Autodesk Inventor part; units mm, degrees
ref_plane "YZ Plane" through (0, 0, 0) normal (1, 0, 0) x (0, 1, 0)
ref_plane "XZ Plane" through (0, 0, 0) normal (0, 1, 0) x (-1, 0, 0)
ref_plane "XY Plane" through (0, 0, 0) normal (0, 0, 1) x (1, 0, 0)
sketch "Sketch4" plane through (0, 0, 0) normal (0, 1, 0) x (-1, 0, 0)
  line L0 (-50.8, 38.1) -> (-50.8, -38.1)
  line L1 (-50.8, -38.1) -> (50.8, -38.1)
  line L2 (50.8, -38.1) -> (50.8, 38.1)
  line L3 (50.8, 38.1) -> (-50.8, 38.1)
  line L4 (-50.8, 38.1) -> (50.8, -38.1) construction
  line L5 (-50.8, -38.1) -> (50.8, 38.1) construction
  point P0 (0, 0)
  dimension "d14" = 76.2
  dimension "d15" = 101.6
extrude "Extrusion4" add sketch "Sketch4" along normal blind 6.35
sketch "Sketch6" plane through (0, 6.35, 0) normal (0, 1, 0) x (1, 0, 0)
  line L0 (-50.8, 38.1) -> (-50.8, -38.1) construction
  line L1 (-50.8, 0) -> (50.8, 0) construction
  line L2 (50.8, -38.1) -> (50.8, 38.1) construction
  line L3 (-50.8, -12.7) -> (-25.4, -12.7)
  line L4 (-25.4, -12.7) -> (-25.4, 12.7)
  line L5 (-25.4, 12.7) -> (-50.8, 12.7)
  line L6 (-50.8, 12.7) -> (-50.8, -12.7)
  line L7 (-50.8, -12.7) -> (-25.4, 12.7) construction
  line L8 (-25.4, -12.7) -> (-50.8, 12.7) construction
  line L9 (-47.625, -9.525) -> (-28.575, -9.525)
  line L10 (-28.575, -9.525) -> (-28.575, 9.525)
  line L11 (-28.575, 9.525) -> (-47.625, 9.525)
  line L12 (-47.625, 9.525) -> (-47.625, -9.525)
  line L13 (-47.625, -9.525) -> (-28.575, 9.525) construction
  line L14 (-28.575, -9.525) -> (-47.625, 9.525) construction
  line L15 (50.8, 38.1) -> (-50.8, 38.1) construction
  line L16 (0, 38.1) -> (0, -38.1) construction
  line L17 (-50.8, -38.1) -> (50.8, -38.1) construction
  line L18 (50.8, -12.7) -> (25.4, -12.7)
  line L19 (25.4, -12.7) -> (25.4, 12.7)
  line L20 (25.4, 12.7) -> (50.8, 12.7)
  line L21 (50.8, 12.7) -> (50.8, -12.7)
  line L22 (47.625, -9.525) -> (28.575, -9.525)
  line L23 (28.575, -9.525) -> (28.575, 9.525)
  line L24 (28.575, 9.525) -> (47.625, 9.525)
  line L25 (47.625, 9.525) -> (47.625, -9.525)
  point P0 (0, 0)
  point P1 (-38.1, 0)
  dimension "d18" = 25.4
  dimension "d19" = 3.175
extrude "Extrusion5" add sketch "Sketch6" along normal blind 298.45
sketch "Sketch7" plane through (-50.8, 0, -38.1) normal (-1, 0, 0) x (0, 0, 1)
  line L0 (25.4, 304.8) -> (50.8, 304.8) construction
  line L1 (38.1, 304.8) -> (38.1, 0) construction
  point P0 (38.1, 279.4)
  point P1 (38.1, 58.674)
  dimension "d22" = 25.4
  dimension "d24" = 246.126
hole "Hole1" at (-50.8, 279.4, 0) at (-50.8, 58.674, 0) direction (1, 0, 0) diameter 6.35 end through all
equation "\"d14\" = supportLength"
equation "\"d15\" = supportWidth"
equation "\"d16\" = supportFloorThickness"
equation "\"d18\" = supportTubingSize"
equation "\"d19\" = supportWallTubingThickness"
equation "\"d20\" = supportTubingHeight"
equation "\"d25\" = supportAxelDiam"
equation "\"supportHeight\" = 304.8"
equation "\"supportWidth\" = 101.6"
equation "\"supportLength\" = 76.2"
equation "\"supportSideHoleDiam\" = 6.35"
equation "\"supporttTopWidth\" = 25.4"
equation "\"supportSupportWidth\" = 101.6"
equation "\"supportSupportPullyHeight\" = 127"
equation "\"supportWallTubingThickness\" = 3.175"
equation "\"supportFloorThickness\" = 6.35"
equation "\"supportTubingHeight\" = supportHeight - supportFloorThickness"
equation "\"supportTubingSize\" = 25.4"
equation "\"supportAxelDistanceFromTop\" = 25.4"
equation "\"supportPulleyAxelDistanceFromTop\" = 246.126"
equation "\"supportAxelDiam\" = 6.35"
properties part number "catapultArmSupportStructure"
The listing builds one solid part. Answer for the finished solid, in the listing's coordinates (mm). A direction names the side the tool comes from. Coordinates: 2 decimals unless noted, no trailing zeros. Order: outer loops, then holes, each group sorted by start corner. A loop starts at its lowest first (then second) coordinate and runs counter-clockwise, first axis right, second up.
Q1. A cutting plane is placed at A-A, the plane y = 188.5. Write down the section's boundary in (x, z) (3 decimals), and give its area (3 significant figures).
Q2. Which of the six approach directions +Z, -Z, +X, -X, +Y, -Y give full straight-line access (tool end or side, diameter ignored) to faces 4 (the face through (25.4, 153, 0)), 5 (the face through (38, 153, 12.7)), 6 (the face through (38, 6.35, 0))?
Q3. For a pull along X with two mould halves and no side action, classify faces 1 (the face through (-28.575, 153, 0)), 2 (the face through (50.8, 140, 3)), 3 (the face through (-38, 153, -12.7)) as pulls with the +X half, pulls with the -X half, needs draft (parallel to the pull), parting line crosses it, or undercut.
Q4. A cutting plane is placed at C-C, the plane y = 279.4. State how many separate pieces and enclosed holes the cut face has, and give its area (3 significant figures).
Q5. A cutting plane is placed at B-B, the plane x = 34. Write down the section's boundary in (y, z) (3 decimals).
Q6. Given P1, Ø5.5, axis at y = 279.4, z = 0, coming from the -X side; P2, Ø9.5, axis at x = 37, y = 86.5, coming from the -Z side; P3, Ø2, axis at x = -33, z = 23.5, coming from the +Y side; P4, Ø5.5, axis at x = 40, y = 87, coming from the +Z side, each flat-ended and moving along its own axis, determine where each tip first touches the part or whether it passes through.
Q7. Consider line 1 (X direction, y = 62.5, z = 1.5) (3 decimals); line 2 (Y direction, x = 27, z = 0) (3 decimals); line 3 (Z direction, x = -29, y = 226) (3 decimals). Determine where each line is inside the solid, lowest interval first.
Answers follow:
1. outline: (-50.8, -12.7) - (-25.4, -12.7) - (-25.4, 12.7) - (-50.8, 12.7) - close; (25.4, -12.7) - (50.8, -12.7) - (50.8, 12.7) - (25.4, 12.7) - close; hole (-47.625, -9.525) - (-28.575, -9.525) - (-28.575, 9.525) - (-47.625, 9.525) - close; hole (28.575, -9.525) - (47.625, -9.525) - (47.625, 9.525) - (28.575, 9.525) - close
1. area: 565 mm2
2. face 4: +Z, -Z, +Y
2. face 5: +Z, +X, -X, +Y
2. face 6: +Y
3. face 1: undercut
3. face 2: pulls with the +X half
3. face 3: needs draft
4. separate pieces: 4
4. enclosed holes: 0
4. area: 484 mm2
5. outline: (0, -38.1) - (6.35, -38.1) - (6.35, -12.7) - (304.8, -12.7) - (304.8, -9.525) - (6.35, -9.525) - (6.35, 9.525) - (304.8, 9.525) - (304.8, 12.7) - (6.35, 12.7) - (6.35, 38.1) - (0, 38.1) - close
6. P1: passes through
6. P2: stops at z = -12.7
6. P3: stops at y = 6.35
6. P4: stops at z = 12.7
7. line 1: x = -50.8 to -47.625, -28.575 to -25.4, 25.4 to 28.575, 47.625 to 50.8
7. line 2: y = 0 to 55.499, 61.849 to 276.225, 282.575 to 304.8
7. line 3: z = -12.7 to -9.525, 9.525 to 12.7
